Answer from the drawing. Dimensions are ordinates in mm from the lowest x, y and z of the part. A direction names the side the tool comes from. Round coordinates to 2 decimals unless told otherwise and drop trailing zeros. Order: outer loops, then holes, each group sorted by start corner. A loop starts at its lowest first (then second) coordinate and runs counter-clockwise, first axis right, second up. Notation, with made-up numbers: M 1.5,-17 L 57.5,-17 A6 cw 57.5,-11 Z; hole C 29,40.25 d4. An arc over 180 degrees is marked long. Answer as a JSON object with one key per item and string values. Group by question number.
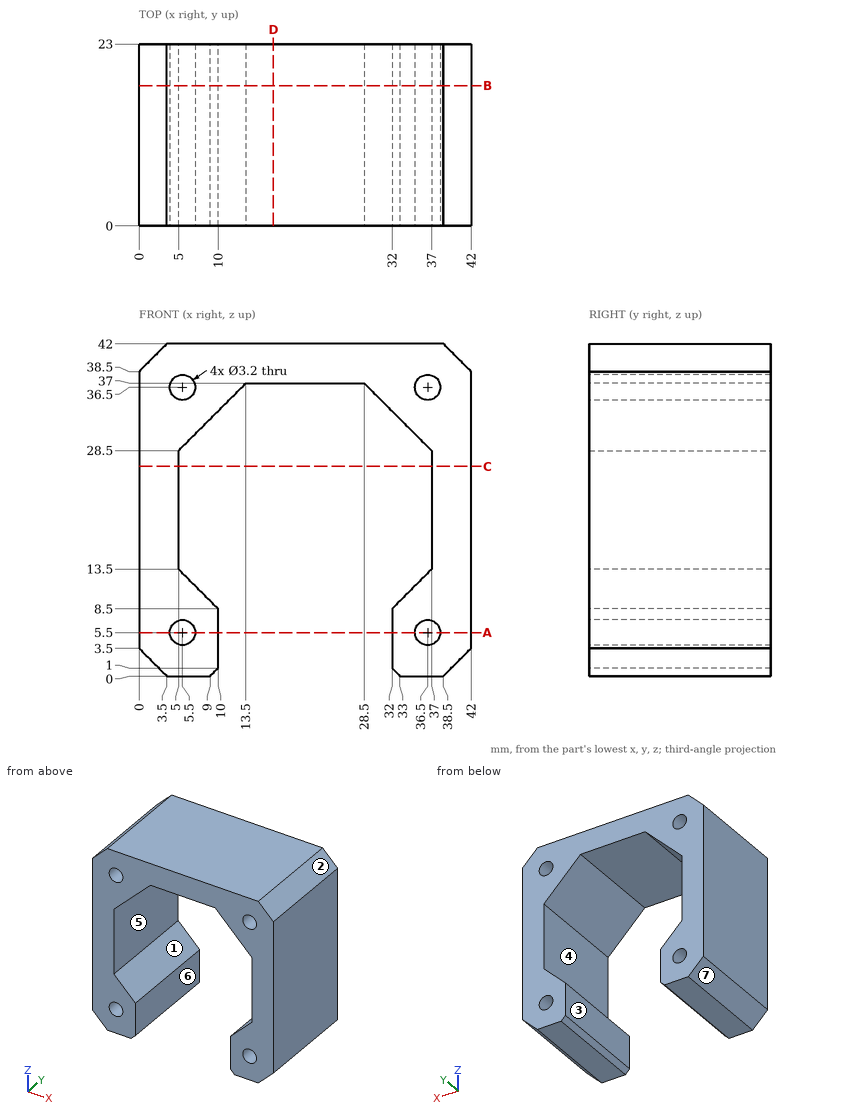
Item 1: Find section D-D (x = 17). Give the vertices of the cut face in (y, z).
Item 2: Find section B-B (y = 17.75). Give the vertices of the cut face in (x, z), and give its area (3 significant figures).
Item 3: A tool of negligible diameter and unlimited length cuts with its end or side. For the marked faces 1, 2 and 3, from which of +Z, -Z, +X, -X, +Y, -Y can it reach the whole face along a straight path? Write none if from no direction.
Item 4: Each of these flat-tipped pins is pushed along its axis until it touches: pin 1 (2.5 mm diameter, centred on x = 36.5, z = 5.5, fed in from +Y); pin 2 (4.5 mm diameter, centred on x = 20, y = 8, fed in from -Z); pin 3 (1.5 mm diameter, centred on x = 11, y = 12.5, fed in from -Z). Where does it stop, or does it pass through?
Item 5: Find section C-C (z = 26.5). Give the vertices of the cut face in (x, y).
Item 6: The mould has two halves that part along Z. Classify the marked faces 4, 5, 6 and 7: +Z half, -Z half, draft (parallel to the pull), parting line (faces both ways), or undercut.
Item 7: Find section A-A (z = 5.5). Give the vertices of the cut face in (x, y), and give its area (3 significant figures).
Item 8: Consider L1, parallel to Z at x = 36.5, y = 18; L2, parallel to Z at x = 33.5, y = 2.5; L3, parallel to X at y = 16.5, z = 6. Determine where each line is inside the solid, lowest interval first.
Responses:
{
 "1": {"outline": "M 0,37 L 23,37 L 23,42 L 0,42 Z"},
 "2": {"outline": "M 0,3.5 L 3.5,0 L 9,0 L 10,1 L 10,8.5 L 5,13.5 L 5,28.5 L 13.5,37 L 28.5,37 L 37,28.5 L 37,13.5 L 32,8.5 L 32,1 L 33,0 L 38.5,0 L 42,3.5 L 42,38.5 L 38.5,42 L 3.5,42 L 0,38.5 Z; hole C 5.5,5.5 d3.2; hole C 5.5,36.5 d3.2; hole C 36.5,5.5 d3.2; hole C 36.5,36.5 d3.2", "area": "705 mm^2"},
 "3": {"face 1": "+Y, -Y", "face 2": "+Z, +X, +Y, -Y", "face 3": "-Z, +Y, -Y"},
 "4": {"pin 1": "passes through", "pin 2": "stops at z = 37", "pin 3": "stops at z = 33.75"},
 "5": {"outline": "M 0,0 L 5,0 L 5,23 L 0,23 Z; M 37,0 L 42,0 L 42,23 L 37,23 Z"},
 "6": {"face 4": "undercut", "face 5": "undercut", "face 6": "draft", "face 7": "-Z half"},
 "7": {"outline": "M 0,0 L 3.9,0 L 3.9,23 L 0,23 Z; M 7.1,0 L 10,0 L 10,23 L 7.1,23 Z; M 32,0 L 34.9,0 L 34.9,23 L 32,23 Z; M 38.1,0 L 42,0 L 42,23 L 38.1,23 Z", "area": "313 mm^2"},
 "8": {"L1": "z = 0 to 3.9, 7.1 to 13, 29 to 34.9, 38.1 to 42", "L2": "z = 0 to 10, 32 to 42", "L3": "x = 0 to 3.98, 7.02 to 10, 32 to 34.98, 38.02 to 42"}
}
